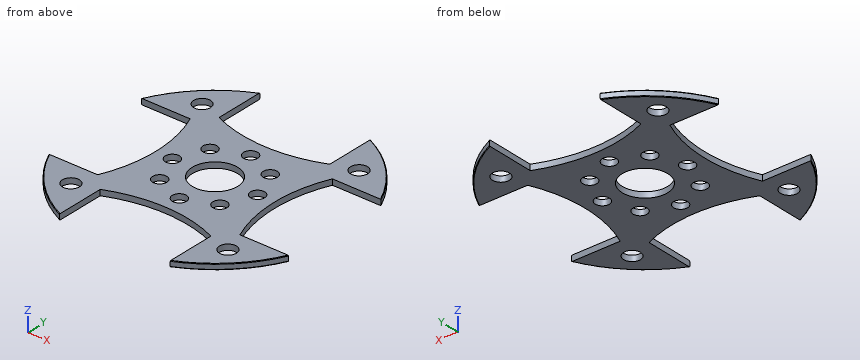
from build123d import *

# Parameters (mm, degrees)
SKETCH_1_R      = 4
SKETCH_1_R_2    = 1.25
SKETCH_1_R_3    = 1.5
EXTRUDE_1_DEPTH = 1
FILLET_1_R      = 0.1


with BuildPart() as part:
    # Эскиз1 → Бобышка-Вытянуть1 (new body)
    with BuildSketch(Plane.XY):
        with BuildLine():
            Line((21.106870919, 9.75), (12.523623513, 9.75))
            ThreePointArc((12.523623513, 9.75), (10.5, 0), (12.523623513, -9.75))
            Line((12.523623513, -9.75), (21.106870919, -9.75))
            ThreePointArc((21.106870919, -9.75), (16.440232663, -16.440232663), (9.75, -21.106870919))
            Line((9.75, -21.106870919), (9.75, -12.523623513))
            ThreePointArc((9.75, -12.523623513), (0, -10.5), (-9.75, -12.523623513))
            Line((-9.75, -12.523623513), (-9.75, -21.106870919))
            ThreePointArc((-9.75, -21.106870919), (-16.440232663, -16.440232663), (-21.106870919, -9.75))
            Line((-21.106870919, -9.75), (-12.523623513, -9.75))
            ThreePointArc((-12.523623513, -9.75), (-10.5, 0), (-12.523623513, 9.75))
            Line((-12.523623513, 9.75), (-21.106870919, 9.75))
            ThreePointArc((-21.106870919, 9.75), (-16.440232663, 16.440232663), (-9.75, 21.106870919))
            Line((-9.75, 21.106870919), (-9.75, 12.523623513))
            ThreePointArc((-9.75, 12.523623513), (0, 10.5), (9.75, 12.523623513))
            Line((9.75, 12.523623513), (9.75, 21.106870919))
            ThreePointArc((9.75, 21.106870919), (16.440232663, 16.440232663), (21.106870919, 9.75))
        make_face()
        Circle(SKETCH_1_R, mode=Mode.SUBTRACT)
        with Locations((0, 7.5)):
            Circle(SKETCH_1_R_2, mode=Mode.SUBTRACT)
        with Locations((5.303300859, 5.303300859)):
            Circle(SKETCH_1_R_2, mode=Mode.SUBTRACT)
        with Locations((7.5, 0)):
            Circle(SKETCH_1_R_2, mode=Mode.SUBTRACT)
        with Locations((5.303300859, -5.303300859)):
            Circle(SKETCH_1_R_2, mode=Mode.SUBTRACT)
        with Locations((0, -7.5)):
            Circle(SKETCH_1_R_2, mode=Mode.SUBTRACT)
        with Locations((-5.303300859, -5.303300859)):
            Circle(SKETCH_1_R_2, mode=Mode.SUBTRACT)
        with Locations((-7.5, 0)):
            Circle(SKETCH_1_R_2, mode=Mode.SUBTRACT)
        with Locations((-5.303300859, 5.303300859)):
            Circle(SKETCH_1_R_2, mode=Mode.SUBTRACT)
        with Locations((13.825687912, 13.825687912)):
            Circle(SKETCH_1_R_3, mode=Mode.SUBTRACT)
        with Locations((13.825687912, -13.825687912)):
            Circle(SKETCH_1_R_3, mode=Mode.SUBTRACT)
        with Locations((-13.825687912, -13.825687912)):
            Circle(SKETCH_1_R_3, mode=Mode.SUBTRACT)
        with Locations((-13.825687912, 13.825687912)):
            Circle(SKETCH_1_R_3, mode=Mode.SUBTRACT)
    extrude(amount=EXTRUDE_1_DEPTH)

    # Скругление1
    fillet_1_edges = [part.edges().sort_by_distance(p)[0] for p in [
        (16.440232663, 16.440232663, 1),
        (16.440232663, -16.440232663, 0),
        (-16.440232663, -16.440232663, 0),
        (-16.440232663, 16.440232663, 0),
        (16.440232663, 16.440232663, 0),
        (-16.440232663, 16.440232663, 1),
        (-16.440232663, -16.440232663, 1),
        (16.440232663, -16.440232663, 1),
    ]]
    fillet(fillet_1_edges, radius=FILLET_1_R)


solid = part.part
Source: CAD feature listing. Evaluate the final solid. Frame: model axes, mm. Coordinates: 2 decimals unless noted, no trailing zeros. Order: outer loops, then holes, each group sorted by start corner. A loop starts at its lowest first (then second) coordinate and runs counter-clockwise, first axis right, second up.
Item 1: Cut plane A-A (x = 0). Return loops of the section in (y, z).
Output values:
outline: (-10.5, 0) - (-8.75, 0) - (-8.75, 1) - (-10.5, 1) - close; (-6.25, 0) - (-4, 0) - (-4, 1) - (-6.25, 1) - close; (4, 0) - (6.25, 0) - (6.25, 1) - (4, 1) - close; (8.75, 0) - (10.5, 0) - (10.5, 1) - (8.75, 1) - close
Item 2: Cut plane D-D (z = 0.4). Count the separate pieces of the cut face and the enclosed holes in it, plus the area to 3 significant figures.
Output values:
separate pieces: 1
enclosed holes: 13
area: 692 mm2
Item 3: First-contact query: P1, Ø1.8, axis at x = 13.83, y = 13.83, coming from the +Z side; P2, Ø13, axis at x = 0, y = 0, coming from the -Z side. Flat tips, straight axial feed; report the tip coordinate or a pass-through.
Output values:
P1: passes through
P2: stops at z = 0
Item 4: Material intervals for line 1 (Y direction, x = 14.5, z = 0.4); line 2 (X direction, y = 14, z = 0.35); line 3 (X direction, y = -1, z = 0.55), sorted ascending.
Output values:
line 1: y = -18.17 to -15.17, -12.49 to -9.75, 9.75 to 12.49, 15.17 to 18.17
line 2: x = -18.56 to -15.32, -12.34 to -9.75, 9.75 to 12.34, 15.32 to 18.56
line 3: x = -10.52 to -8.25, -6.75 to -3.87, 3.87 to 6.75, 8.25 to 10.52
Item 5: Cut plane C-C (y = -7.5). Return loops of the section in (x, z).
Output values:
outline: (-11.68, 0) - (-1.25, 0) - (-1.25, 1) - (-11.68, 1) - close; (1.25, 0) - (11.68, 0) - (11.68, 1) - (1.25, 1) - close
